```python
from build123d import *

# Parameters (mm, degrees)
BOSS_EXTRUDE1_DEPTH = 6
SKETCH2_R           = 1.5
CUT_EXTRUDE1_DEPTH  = 10
SKETCH3_R           = 3
SKETCH3_R_2         = 1.5
CUT_EXTRUDE2_DEPTH  = 3


with BuildPart() as part:
    # Sketch1 → Boss-Extrude1 (new body)
    with BuildSketch(Plane(origin=(0, 0, 0), x_dir=(1, 0, 0), z_dir=(0, 1, 0))):
        with BuildLine():
            Line((70, -99), (70, 99))
            ThreePointArc((70, 99), (68.242640687, 103.242640687), (64, 105))
            Line((64, 105), (-64, 105))
            ThreePointArc((-64, 105), (-68.242640687, 103.242640687), (-70, 99))
            Line((-70, 99), (-70, -99))
            ThreePointArc((-70, -99), (-68.242640687, -103.242640687), (-64, -105))
            Line((-64, -105), (64, -105))
            ThreePointArc((64, -105), (68.242640687, -103.242640687), (70, -99))
        make_face()
    extrude(amount=BOSS_EXTRUDE1_DEPTH)

    # Sketch2 → Cut-Extrude1 (cut)
    with BuildSketch(Plane(origin=(0, 6, 0), x_dir=(1, 0, 0), z_dir=(0, 1, 0))):
        with Locations(Location((-64, -82.5, 0), (0, 0, 270))):
            Circle(SKETCH2_R)
        with Locations(Location((-64, -52.5, 0), (0, 0, 270))):
            Circle(SKETCH2_R)
        with Locations(Location((-64, -22.5, 0), (0, 0, 270))):
            Circle(SKETCH2_R)
        with Locations(Location((-64, 7.5, 0), (0, 0, 270))):
            Circle(SKETCH2_R)
        with Locations(Location((-64, 37.5, 0), (0, 0, 270))):
            Circle(SKETCH2_R)
        with Locations(Location((-64, 67.5, 0), (0, 0, 270))):
            Circle(SKETCH2_R)
        with Locations(Location((64, -67.5, 0), (0, 0, 270))):
            Circle(SKETCH2_R)
        with Locations(Location((64, -37.5, 0), (0, 0, 270))):
            Circle(SKETCH2_R)
        with Locations(Location((64, -7.5, 0), (0, 0, 270))):
            Circle(SKETCH2_R)
        with Locations(Location((64, 22.5, 0), (0, 0, 270))):
            Circle(SKETCH2_R)
        with Locations(Location((64, 52.5, 0), (0, 0, 270))):
            Circle(SKETCH2_R)
        with Locations(Location((64, 82.5, 0), (0, 0, 270))):
            Circle(SKETCH2_R)
    extrude(amount=-CUT_EXTRUDE1_DEPTH, mode=Mode.SUBTRACT)

    # Sketch3 → Cut-Extrude2 (cut)
    # profile 1 of 12: a face of its own
    with BuildSketch(Plane(origin=(0, 6, 0), x_dir=(1, 0, 0), z_dir=(0, 1, 0))):
        with Locations(Location((-64, -82.5, 0), (0, 0, 270))):
            Circle(SKETCH3_R)
        with Locations(Location((-64, -82.5, 0), (0, 0, 270))):
            Circle(SKETCH3_R_2, mode=Mode.SUBTRACT)
    # profile 2 of 12: a face of its own
    with BuildSketch(Plane(origin=(0, 6, 0), x_dir=(1, 0, 0), z_dir=(0, 1, 0))):
        with Locations(Location((-64, -52.5, 0), (0, 0, 270))):
            Circle(SKETCH3_R)
    # profile 3 of 12: a face of its own
    with BuildSketch(Plane(origin=(0, 6, 0), x_dir=(1, 0, 0), z_dir=(0, 1, 0))):
        with Locations(Location((-64, -22.5, 0), (0, 0, 270))):
            Circle(SKETCH3_R)
    # profile 4 of 12: a face of its own
    with BuildSketch(Plane(origin=(0, 6, 0), x_dir=(1, 0, 0), z_dir=(0, 1, 0))):
        with Locations(Location((-64, 7.5, 0), (0, 0, 270))):
            Circle(SKETCH3_R)
    # profile 5 of 12: a face of its own
    with BuildSketch(Plane(origin=(0, 6, 0), x_dir=(1, 0, 0), z_dir=(0, 1, 0))):
        with Locations(Location((-64, 37.5, 0), (0, 0, 270))):
            Circle(SKETCH3_R)
    # profile 6 of 12: a face of its own
    with BuildSketch(Plane(origin=(0, 6, 0), x_dir=(1, 0, 0), z_dir=(0, 1, 0))):
        with Locations(Location((-64, 67.5, 0), (0, 0, 270))):
            Circle(SKETCH3_R)
    # profile 7 of 12: a face of its own
    with BuildSketch(Plane(origin=(0, 6, 0), x_dir=(1, 0, 0), z_dir=(0, 1, 0))):
        with Locations(Location((64, -67.5, 0), (0, 0, 270))):
            Circle(SKETCH3_R)
        with Locations(Location((64, -67.5, 0), (0, 0, 270))):
            Circle(SKETCH3_R_2, mode=Mode.SUBTRACT)
    # profile 8 of 12: a face of its own
    with BuildSketch(Plane(origin=(0, 6, 0), x_dir=(1, 0, 0), z_dir=(0, 1, 0))):
        with Locations(Location((64, -37.5, 0), (0, 0, 270))):
            Circle(SKETCH3_R)
        with Locations(Location((64, -37.5, 0), (0, 0, 270))):
            Circle(SKETCH3_R_2, mode=Mode.SUBTRACT)
    # profile 9 of 12: a face of its own
    with BuildSketch(Plane(origin=(0, 6, 0), x_dir=(1, 0, 0), z_dir=(0, 1, 0))):
        with Locations(Location((64, -7.5, 0), (0, 0, 270))):
            Circle(SKETCH3_R)
        with Locations(Location((64, -7.5, 0), (0, 0, 270))):
            Circle(SKETCH3_R_2, mode=Mode.SUBTRACT)
    # profile 10 of 12: a face of its own
    with BuildSketch(Plane(origin=(0, 6, 0), x_dir=(1, 0, 0), z_dir=(0, 1, 0))):
        with Locations(Location((64, 22.5, 0), (0, 0, 270))):
            Circle(SKETCH3_R)
        with Locations(Location((64, 22.5, 0), (0, 0, 270))):
            Circle(SKETCH3_R_2, mode=Mode.SUBTRACT)
    # profile 11 of 12: a face of its own
    with BuildSketch(Plane(origin=(0, 6, 0), x_dir=(1, 0, 0), z_dir=(0, 1, 0))):
        with Locations(Location((64, 52.5, 0), (0, 0, 270))):
            Circle(SKETCH3_R)
        with Locations(Location((64, 52.5, 0), (0, 0, 270))):
            Circle(SKETCH3_R_2, mode=Mode.SUBTRACT)
    # profile 12 of 12: a face of its own
    with BuildSketch(Plane(origin=(0, 6, 0), x_dir=(1, 0, 0), z_dir=(0, 1, 0))):
        with Locations(Location((64, 82.5, 0), (0, 0, 270))):
            Circle(SKETCH3_R)
        with Locations(Location((64, 82.5, 0), (0, 0, 270))):
            Circle(SKETCH3_R_2, mode=Mode.SUBTRACT)
    extrude(amount=-CUT_EXTRUDE2_DEPTH, mode=Mode.SUBTRACT)


solid = part.part
```
Build history of the part. All positions in model axes, mm. A direction names the side the tool comes from. Give positions to 0.01 mm unless a question says otherwise; leave off trailing zeros.
Item 1: Flat gauge pins, fed straight in: pin 1 (9.5 mm diameter, centred on x = 64, z = 37.5, fed in from -Y); pin 2 (2.5 mm diameter, centred on x = 64, z = -22.5, fed in from -Y); pin 3 (1.8 mm diameter, centred on x = -65.5, z = 23.5, fed in from +Y). Where does each tip first touch, or does it go through?
Answers follow:
pin 1: stops at y = 0
pin 2: passes through
pin 3: stops at y = 3
Item 2: Drill centre lines: line 1 (X direction, y = 5, z = 67.5); line 2 (X direction, y = 1.15, z = -7.5). Where is each one in solid material? Low to high.
Answers follow:
line 1: x = -70 to 61, 67 to 70
line 2: x = -70 to -65.5, -62.5 to 70
Item 3: Pull direction Z, two halves, no side cores. Call faces 1 (the face through (-61.47, 4.52, -5.89)), 2 (the face through (68.289, 2.958, -103.196)), 3 (the face through (-1, 3, 105)): released by +Z, released by -Z, zero draft, split by the parting line, or undercut.
Answers follow:
face 1: undercut
face 2: released by -Z
face 3: released by +Z
Item 4: Which spindle directions (+Z, -Z, +X, -X, +Y, -Y) get a long thin tool onto all of the face, cutting with end or side? Do faces 4 (the face through (70, 3, 1)), 5 (the face through (64.1, 4.5, -55.5)). Say none if no direction does.
Answers follow:
face 4: +Z, -Z, +X, +Y, -Y
face 5: +Y
